Check sheet for the drawn part. Datum: minimum x, y, z corner. Units: mm. Round coordinates to 2 decimals unless told otherwise and drop trailing zeros. Write each loop counter-clockwise with the first axis right and the second up, starting at its lowest first coordinate (ties: lowest second). Pieces come first, ordered by that corner, then holes. Notation, with made-up numbers: (70.25, 5) -> (83.25, 5) arc R25 cw to (83.25, 22) -> close; hole circle Ø8 at (48, 55). An arc over 180 degrees is marked (long way). One line per item, written item: value.
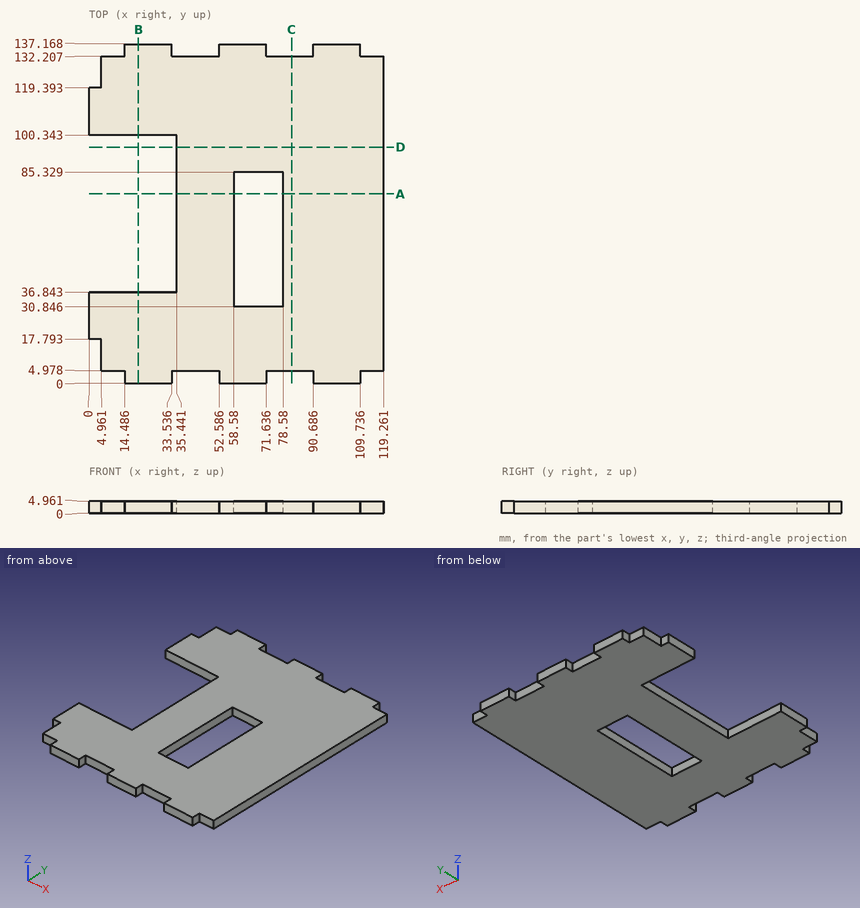
Item 1: Sectioned sample at C-C on x = 82. Enter the section's corners in (y, z), and give its area (3 significant figures).
Answer:
outline: (4.98, 0) -> (132.21, 0) -> (132.21, 4.96) -> (4.98, 4.96) -> close
area: 631 mm^2
Item 2: Sectioned sample at B-B on x = 20. Enter the section's corners in (y, z).
Answer:
outline: (0, 0) -> (36.84, 0) -> (36.84, 4.96) -> (0, 4.96) -> close; (100.34, 0) -> (137.17, 0) -> (137.17, 4.96) -> (100.34, 4.96) -> close
Item 3: Depth check by flat-ended pin: P1, Ø1.5, axis at x = 35.5, z = 4, coming from the -Y side; P2, Ø2.5, axis at y = 134.5, z = 2, coming from the +X side; P3, Ø2, axis at y = 47.5, z = 1.5, coming from the -X side. Enter the tip coordinate at first touch or a pass-through.
Answer:
P1: stops at y = 4.98
P2: stops at x = 109.74
P3: stops at x = 35.44
Item 4: Sectioned sample at D-D on y = 95.5. Enter the section's corners in (x, z), and give its area (3 significant figures).
Answer:
outline: (35.44, 0) -> (119.26, 0) -> (119.26, 4.96) -> (35.44, 4.96) -> close
area: 416 mm^2
Item 5: Thickness scan on line 1 (X direction, y = 52, z = 4.2); line 2 (Y direction, x = 13, z = 4.7); line 3 (Y direction, x = 69, z = 1.95). Record the ranges inside material, lowest first.
Answer:
line 1: x = 35.44 to 58.58, 78.58 to 119.26
line 2: y = 4.98 to 36.84, 100.34 to 132.21
line 3: y = 0 to 30.85, 85.33 to 137.17
Item 6: Sectioned sample at A-A on y = 76.5. Enter the section's corners in (x, z).
Answer:
outline: (35.44, 0) -> (58.58, 0) -> (58.58, 4.96) -> (35.44, 4.96) -> close; (78.58, 0) -> (119.26, 0) -> (119.26, 4.96) -> (78.58, 4.96) -> close
